The model under review builds one solid part; all positions refer to its coordinate system, in mm. Face numbers are marked on the shaded views. A direction names the side the tool comes from. Coordinates: 2 decimals unless noted, no trailing zeros. Loops run counter-clockwise (first coordinate to the right, second up) from the corner with the lowest first, then second, coordinate; pieces in that order, holes last. Notation, with made-up numbers: M 71,82.25 L 82,82.25 A16 ccw 82,102.25 Z; hole C -2,39 d7. An arc over 180 degrees is marked long. Return JSON: item names as keys, results as strings.
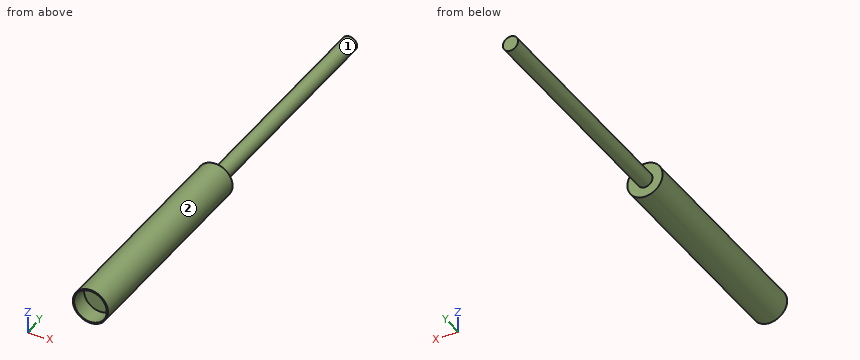
```python
from build123d import *

# Parameters (mm, degrees)
F0_R     = 25.4
F1_DEPTH = 317.5
F2_R     = 23.622
F3_DEPTH = 25.4
F4_R     = 10.922
F5_DEPTH = 342.9


with BuildPart() as f1:
    # F0 (on Front) → F1 (new body)
    with BuildSketch(Plane.XZ):
        Circle(F0_R)
    extrude(amount=F1_DEPTH)

    # F2 (on face) → F3 (cut)
    with BuildSketch(Plane.XZ.offset(317.5)):
        Circle(F2_R)
    extrude(amount=-F3_DEPTH, mode=Mode.SUBTRACT)

    # F4 (on Front) → F5 (join)
    with BuildSketch(Plane.XZ):
        Circle(F4_R)
    extrude(amount=-F5_DEPTH)


solid = f1.part
```
1. Add section B-B on x = 0. Give the boundary of the cut face in (y, z).
Check values:
{"outline": "M -317.5,-25.4 L 0,-25.4 L 0,-10.92 L 342.9,-10.92 L 342.9,10.92 L 0,10.92 L 0,25.4 L -317.5,25.4 L -317.5,23.62 L -292.1,23.62 L -292.1,-23.62 L -317.5,-23.62 Z"}
2. To check wall thickness, follow line 1 (Z direction, x = 0, y = -306); line 2 (Y direction, x = -12.5, z = -22); line 3 (Y direction, x = -15.5, z = -6). State the ranges of each line that lie inside material, in increasing order.
Check values:
{"line 1": "-25.4 to -23.62, 23.62 to 25.4", "line 2": "-317.5 to 0", "line 3": "-292.1 to 0"}
3. Insertion check: pin 1 Ø10 at (x, y) = (9.5, 134.5) entering from +Z; pin 2 Ø10 at (y, z) = (151.5, 2) entering from +X; pin 3 Ø1.5 at (x, z) = (15.5, 1) entering from -Y. Each pin has a flat end and moves straight along its axis. Give the tip position at first contact, or say it passes through.
Check values:
{"pin 1": "z = 9.95", "pin 2": "x = 10.92", "pin 3": "y = -292.1"}
4. Machinability: for the marked faces 1 and 2, which of the approach directions +Z, -Z, +X, -X, +Y, -Y give a long, thin tool a straight path to every point of the face, cutting with its end or side? Answer none if there is none.
Check values:
{"face 1": "+Y", "face 2": "+Y, -Y"}
5. Add section D-D on y = -70. Give the boundary of the cut face in (x, z), plus the area to 3 significant figures.
Check values:
{"outline": "C 0,0 d50.8", "area": "2,030 mm²"}
6. Add section A-A on z = 0. Give the boundary of the cut face in (x, y).
Check values:
{"outline": "M -25.4,-317.5 L -23.62,-317.5 L -23.62,-292.1 L 23.62,-292.1 L 23.62,-317.5 L 25.4,-317.5 L 25.4,0 L 10.92,0 L 10.92,342.9 L -10.92,342.9 L -10.92,0 L -25.4,0 Z"}
7. Add section C-C on y = 144.5. Give the boundary of the cut face in (x, z).
Check values:
{"outline": "C 0,0 d21.84"}
